```python
from build123d import *

# Parameters (mm, degrees)
SKETCH_1_W      = 35.6
SKETCH_1_H      = 31.8
EXTRUDE_1_DEPTH = 1
SKETCH_2_W      = 35.6
SKETCH_2_H      = 19.3
EXTRUDE_2_DEPTH = 1.5
SKETCH_3_W      = 8.082791172
SKETCH_3_H      = 1.155308412
EXTRUDE_3_DEPTH = 0.1


with BuildPart() as part:
    # 草图1 → 凸台-拉伸1 (new body)
    with BuildSketch(Plane.XY):
        Rectangle(SKETCH_1_W, SKETCH_1_H)
    extrude(amount=EXTRUDE_1_DEPTH)

    # 草图2 → 凸台-拉伸2 (add)
    with BuildSketch(Plane.XY.offset(1)):
        with Locations((0, 1.25)):
            Rectangle(SKETCH_2_W, SKETCH_2_H)
    extrude(amount=EXTRUDE_2_DEPTH)

    # 草图3 → 凸台-拉伸3 (add)
    with BuildSketch(Plane.XY.offset(2.5)):
        with BuildLine():
            Line((8.23788009, -3.216692679), (5.445549995, -3.216692679))
            ThreePointArc((5.445549995, -3.216692679), (5.091996605, -3.363139288), (4.945549995, -3.716692679))
            Line((4.945549995, -3.716692679), (4.945549995, -4.123155093))
            ThreePointArc((4.945549995, -4.123155093), (5.091996605, -4.476708484), (5.445549995, -4.623155093))
            Line((5.445549995, -4.623155093), (12.934555282, -4.623155093))
            ThreePointArc((12.934555282, -4.623155093), (13.288108672, -4.476708484), (13.434555282, -4.123155093))
            Line((13.434555282, -4.123155093), (13.434555282, -3.716692679))
            ThreePointArc((13.434555282, -3.716692679), (13.288108672, -3.363139288), (12.934555282, -3.216692679))
            Line((12.934555282, -3.216692679), (10.594302392, -3.216692679))
            add(Edge.make_bspline(
                [(10.594302392, -3.216692679), (17.453446302, 3.769231485), (9.416091241, 3.769231485), (1.37873618, 3.769231485), (8.23788009, -3.216692679)],
                knots=[0.54830721, 0.54830721, 0.54830721, 3.141592654, 3.141592654, 5.734878097, 5.734878097, 5.734878097], degree=2, weights=[1, 0.270732248, 1, 0.270732248, 1]))
        make_face()
        with Locations((0, 7.708506432)):
            Rectangle(SKETCH_3_W, SKETCH_3_H)
        with BuildLine():
            Line((-4.945549995, -4.123155093), (-4.945549995, -3.716692679))
            ThreePointArc((-4.945549995, -3.716692679), (-5.091996605, -3.363139288), (-5.445549995, -3.216692679))
            Line((-5.445549995, -3.216692679), (-8.23788009, -3.216692679))
            add(Edge.make_bspline(
                [(-8.23788009, -3.216692679), (-1.37873618, 3.769231485), (-9.416091241, 3.769231485), (-17.453446302, 3.769231485), (-10.594302392, -3.216692679)],
                knots=[0.54830721, 0.54830721, 0.54830721, 3.141592654, 3.141592654, 5.734878097, 5.734878097, 5.734878097], degree=2, weights=[1, 0.270732248, 1, 0.270732248, 1]))
            Line((-10.594302392, -3.216692679), (-12.934555282, -3.216692679))
            ThreePointArc((-12.934555282, -3.216692679), (-13.288108672, -3.363139288), (-13.434555282, -3.716692679))
            Line((-13.434555282, -3.716692679), (-13.434555282, -4.123155093))
            ThreePointArc((-13.434555282, -4.123155093), (-13.288108672, -4.476708484), (-12.934555282, -4.623155093))
            Line((-12.934555282, -4.623155093), (-5.445549995, -4.623155093))
            ThreePointArc((-5.445549995, -4.623155093), (-5.091996605, -4.476708484), (-4.945549995, -4.123155093))
        make_face()
    extrude(amount=EXTRUDE_3_DEPTH)


solid = part.part
```
Can you work these out from the model? Positions are in its coordinate system, mm. A direction names the side the tool comes from. Give positions to 0.01 mm unless a question says otherwise; leave off trailing zeros. Loops run counter-clockwise (first coordinate to the right, second up) from the corner with the lowest first, then second, coordinate; pieces in that order, holes last. Notation, with made-up numbers: M -37,50 L 11,50 A10 ccw 11,55 Z; hole C -3.5,-36.75 d4. An arc over 180 degrees is marked long. Use one line per item in the form item = value. Start each with the question number.
(1) I want a section at C-C, the plane y = -6. Write out the boundary of the cut face in (x, z).
(2) On a 3-axis mill with a long thin cutter (end or side, diameter ignored), from which of +Z, -Z, +X, -X, +Y, -Y can I reach the whole of each face in a straight line? I mean faces 1 (the flat face through (0, -12, 1)), 2 (the flat face through (0, 10.9, 2)), 3 (the flat face through (-0.2, -15.9, 0.5)). Say none if no direction works.
(3) I want a section at D-D, the plane z = 1.9. Write out the boundary of the cut face in (x, y).
(4) Thinking about a two-plate mould opening in X: for faces 4 (the flat face through (-17.8, 0, 1)), 5 (the flat face through (17.8, 0, 1)), 6 (the flat face through (0, 1, 2.5)), 7 (the flat face through (0, 13, 1)), which applies, released by +X, released by -X, zero draft, split by the parting line, or undercut?
(5) Please list where these lines run through material, in increasing order: line 1 (Z direction, x = -8, y = 6); line 2 (Z direction, x = 13, y = -12.5); line 3 (Y direction, x = -12.5, z = 2.4).
(6) I'm going to push flat-ended pins straight in: P1, Ø8, axis at x = -5, y = -12.5, coming from the +Z side; P2, Ø1.5, axis at x = -12.5, y = -9, coming from the +Z side. Where does each tip first touch, or does it pass through?
(7) I want a section at B-B, the plane x = 6. Write out the boundary of the cut face in (y, z).
(8) I want a section at A-A, the plane x = 0. Write out the boundary of the cut face in (y, z).
Worked out:
q1.outline = M -17.8,0 L 17.8,0 L 17.8,2.5 L -17.8,2.5 Z
q2.face_1 = +Z, +X, -X, -Y
q2.face_2 = +Z, +X, -X, +Y
q2.face_3 = +Z, -Z, +X, -X, -Y
q3.outline = M -17.8,-8.4 L 17.8,-8.4 L 17.8,10.9 L -17.8,10.9 Z
q4.face_4 = released by -X
q4.face_5 = released by +X
q4.face_6 = undercut
q4.face_7 = zero draft
q5.line_1 = 0 to 2.5
q5.line_2 = 0 to 1
q5.line_3 = -8.4 to 10.9
q6.P1 = 1
q6.P2 = 2.5
q7.outline = M -15.9,0 L 15.9,0 L 15.9,1 L 10.9,1 L 10.9,2.5 L -3.22,2.5 L -3.22,2.6 L -4.62,2.6 L -4.62,2.5 L -8.4,2.5 L -8.4,1 L -15.9,1 Z
q8.outline = M -15.9,0 L 15.9,0 L 15.9,1 L 10.9,1 L 10.9,2.5 L 8.29,2.5 L 8.29,2.6 L 7.13,2.6 L 7.13,2.5 L -8.4,2.5 L -8.4,1 L -15.9,1 Z
